Model file for the job. Use its own axes, mm. Face numbers are marked on the shaded views. Give positions to 0.01 mm unless a question says otherwise; leave off trailing zeros. Loops run counter-clockwise (first coordinate to the right, second up) from the corner with the lowest first, then second, coordinate; pieces in that order, holes last. Notation, with made-up numbers: M -10,11.5 L 4,11.5 A19 ccw 4,26.5 Z; hole C -39.5,81.5 d2. An arc over 180 degrees is marked long. Answer in a Markdown table with one row per item.
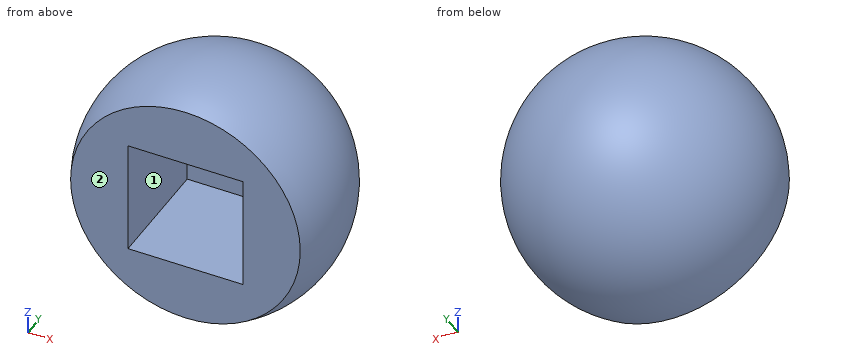
```python
from build123d import *

# Parameters (mm, degrees)
SKETCH2_W          = 8
SKETCH2_H          = 8
CUT_EXTRUDE1_DEPTH = 8


with BuildPart() as part:
    # Sketch1 → Revolve1 (revolve)
    with BuildSketch(Plane.XY, mode=Mode.PRIVATE) as revolve1_sk:
        with BuildLine():
            Line((-8, 0), (0, 0))
            Line((0, 0), (0, 12.94427191))
            ThreePointArc((0, 12.94427191), (-7.60845213, 8.702282018), (-8, 0))
        make_face()
    revolve(revolve1_sk.sketch.rotate(Axis((0, 0, 0), (0, 1, 0)), 180), axis=Axis((0, 0, 0), (0, 1, 0)))

    # Sketch2 → Cut-Extrude1 (cut)
    with BuildSketch(Plane.XZ):
        Rectangle(SKETCH2_W, SKETCH2_H)
    extrude(amount=-CUT_EXTRUDE1_DEPTH, mode=Mode.SUBTRACT)


solid = part.part
```
Q1. Saw through at D-D (y = 7.5). Give the cut face in (x, z), and give its area (3 significant figures).
Reported:
| item | result |
|---|---|
| outline | C 0,0 d16.46; hole M -4,-4 L 4,-4 L 4,4 L -4,4 Z |
| area | 149 mm² |
Q2. Mould opens along X. For the marked faces 1 and 2 say: released by +X, released by -X, zero draft, split by the parting line, or undercut.
Reported:
| item | result |
|---|---|
| face 1 | undercut |
| face 2 | zero draft |
Q3. Saw through at B-B (x = 3.5). Give the cut face in (y, z), and give its area (3 significant figures).
Reported:
| item | result |
|---|---|
| outline | M 0,-7.19 A8.23 ccw long 0,7.19 L 0,4 L 8,4 L 8,-4 L 0,-4 Z |
| area | 106 mm² |
Q4. Drop flat-ended pins along their axis: pin 1 (2 mm diameter, centred on y = 3, z = -7, fed in from +X); pin 2 (2 mm diameter, centred on x = -6.5, z = -6, fed in from +Y); pin 3 (2.5 mm diameter, centred on x = -1.5, y = 2, fed in from +Z). Give the stop position or say it passes through.
Reported:
| item | result |
|---|---|
| pin 1 | x = 6.57 |
| pin 2 | y = 8.29 |
| pin 3 | z = 8.86 |
Q5. Saw through at C-C (z = -1). Give the cut face in (x, y).
Reported:
| item | result |
|---|---|
| outline | M -7.94,0 L -4,0 L -4,8 L 4,8 L 4,0 L 7.94,0 A8.89 ccw long Z |
Q6. Saw through at A-A (y = 5.25). Give the cut face in (x, z).
Reported:
| item | result |
|---|---|
| outline | C 0,0 d17.71; hole M -4,-4 L 4,-4 L 4,4 L -4,4 Z |
Q7. Probe probe 1 along Z at (x, y) = (0.5, 1.75); probe 2 along X at (y, z) = (2.25, 1.25); probe 3 along X at (y, z) = (2.5, 3). List the from-to ranges inside material, lowest first.
Reported:
| item | result |
|---|---|
| probe 1 | -8.64 to -4, 4 to 8.64 |
| probe 2 | -8.68 to -4, 4 to 8.68 |
| probe 3 | -8.29 to -4, 4 to 8.29 |
